Check sheet for the modelled part. Datum: model origin and axes. Units: mm. Face numbers are marked on the shaded views. A direction names the side the tool comes from. Give positions to 0.01 mm unless a question says otherwise; leave off trailing zeros. Write each loop counter-clockwise with the first axis right and the second up, starting at its lowest first coordinate (ties: lowest second). Pieces come first, ordered by that corner, then holes. Notation, with made-up numbers: (-1.5, -38.5) -> (25.5, -38.5) arc R17 ccw to (25.5, -6.5) -> close; hole circle Ø11 at (70, 7.25). An arc over 180 degrees is marked (long way). Use a Markdown table: item, result. Add a question column.
1. Release check for a two-part mould opening along X. For the marked faces 6, 7, 8 and 9 record: released by +X, released by -X, zero draft, split by the parting line, or undercut.
2. Cross-section at B-B (x = 4). Enter the section's corners in (y, z), then the cut area to 3 significant figures.
3. Cross-section at D-D (z = -42). Enter the section's corners in (x, y), then the cut area to 3 significant figures.
4. Set-up check for the marked faces 1, 2, 3, 4 and 5: record each of +Z, -Z, +X, -X, +Y, -Y from which the full face is reachable in a straight line by a thin tool's end or side.
5. Cross-section at A-A (y = 65). Enter the section's corners in (x, z).
6. Scan lines: probe 1 along Y at (x, z) = (-29.5, 48.5); probe 2 along X at (y, z) = (13.5, 1.5); probe 3 along Z at (x, y) = (40, 110). Record each from-to range of solid material in increasing order. Write a range as [from, to].
7. Cross-section at C-C (y = 105). Enter the section's corners in (x, z), then the cut area to 3 significant figures.
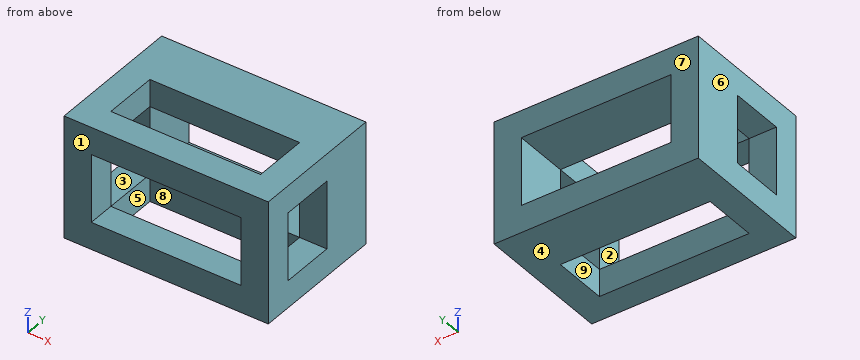
from build123d import *

# Parameters (mm, degrees)
SKETCH1_W           = 190.5
SKETCH1_H           = 114.3
BOSS_EXTRUDE1_DEPTH = 127
SKETCH2_W           = 139.7
SKETCH2_H           = 50.8
CUT_EXTRUDE1_DEPTH  = 196.61710687
SKETCH3_W           = 63.5
SKETCH3_H           = 50.8
CUT_EXTRUDE2_DEPTH  = 236.977483036
SKETCH4_W           = 139.7
SKETCH4_H           = 63.5
CUT_EXTRUDE3_DEPTH  = 169.723694246


with BuildPart() as part:
    # Sketch1 → Boss-Extrude1 (new body)
    with BuildSketch(Plane(origin=(0, 0, 0), x_dir=(1, 0, 0), z_dir=(0, 1, 0))):
        Rectangle(SKETCH1_W, SKETCH1_H)
    extrude(amount=BOSS_EXTRUDE1_DEPTH)

    # Sketch2 → Cut-Extrude1 (cut, through all)
    with BuildSketch(Plane.XY.offset(57.15)):
        with Locations((0, 50.8)):
            Rectangle(SKETCH2_W, SKETCH2_H)
    extrude(amount=-CUT_EXTRUDE1_DEPTH, mode=Mode.SUBTRACT)

    # Sketch3 → Cut-Extrude2 (cut, through all)
    with BuildSketch(Plane(origin=(95.25, 0, 0), x_dir=(0, 0, -1), z_dir=(1, 0, 0))):
        with Locations((0, 50.8)):
            Rectangle(SKETCH3_W, SKETCH3_H)
    extrude(amount=-CUT_EXTRUDE2_DEPTH, mode=Mode.SUBTRACT)

    # Sketch4 → Cut-Extrude3 (cut, through all)
    with BuildSketch(Plane(origin=(0, 127, 0), x_dir=(1, 0, 0), z_dir=(0, 1, 0))):
        Rectangle(SKETCH4_W, SKETCH4_H)
    extrude(amount=-CUT_EXTRUDE3_DEPTH, mode=Mode.SUBTRACT)


solid = part.part
Worked answers:
| question | item | result |
|---|---|---|
| 1 | face 6 | released by -X |
| 1 | face 7 | zero draft |
| 1 | face 8 | undercut |
| 1 | face 9 | undercut |
| 2 | outline | (0, -57.15) -> (25.4, -57.15) -> (25.4, -31.75) -> (0, -31.75) -> close; (0, 31.75) -> (25.4, 31.75) -> (25.4, 57.15) -> (0, 57.15) -> close; (76.2, -57.15) -> (127, -57.15) -> (127, -31.75) -> (76.2, -31.75) -> close; (76.2, 31.75) -> (127, 31.75) -> (127, 57.15) -> (76.2, 57.15) -> close |
| 2 | area | 3,870 mm² |
| 3 | outline | (-95.25, 0) -> (95.25, 0) -> (95.25, 127) -> (-95.25, 127) -> close; hole (-69.85, 25.4) -> (69.85, 25.4) -> (69.85, 76.2) -> (-69.85, 76.2) -> close |
| 3 | area | 17,100 mm² |
| 4 | face 1 | +Z, -Z, +X, -X, -Y |
| 4 | face 2 | +Y, -Y |
| 4 | face 3 | +X, -X |
| 4 | face 4 | -Z, +X, -X, +Y, -Y |
| 4 | face 5 | +Z, -Z |
| 5 | outline | (-95.25, -57.15) -> (-69.85, -57.15) -> (-69.85, -31.75) -> (-95.25, -31.75) -> close; (-95.25, 31.75) -> (-69.85, 31.75) -> (-69.85, 57.15) -> (-95.25, 57.15) -> close; (69.85, -57.15) -> (95.25, -57.15) -> (95.25, -31.75) -> (69.85, -31.75) -> close; (69.85, 31.75) -> (95.25, 31.75) -> (95.25, 57.15) -> (69.85, 57.15) -> close |
| 6 | probe 1 | y = [0, 25.4], [76.2, 127] |
| 6 | probe 2 | x = [-95.25, -69.85], [69.85, 95.25] |
| 6 | probe 3 | z = [-57.15, -31.75], [31.75, 57.15] |
| 7 | outline | (-95.25, -57.15) -> (95.25, -57.15) -> (95.25, 57.15) -> (-95.25, 57.15) -> close; hole (-69.85, -31.75) -> (69.85, -31.75) -> (69.85, 31.75) -> (-69.85, 31.75) -> close |
| 7 | area | 12,900 mm² |
